```python
from build123d import *

# Parameters (mm, degrees)
SKETCH1_W                = 69
SKETCH1_H                = 45
BOSS_EXTRUDE1_DEPTH      = 10
BOSS_EXTRUDE2_DEPTH      = 12
BOSS_EXTRUDE2_DEPTH_BACK = 13
SKETCH5_R                = 19
SKETCH6_R                = 8
CUT_EXTRUDE1_DEPTH       = 146.555831213
FILLET1_R                = 25
FILLET2_R                = 15
FILLET3_R                = 5
FILLET4_R                = 2
FILLET5_R                = 25
FILLET6_R                = 30
SKETCH7_R                = 8
CUT_EXTRUDE2_DEPTH       = 138.282555338


with BuildPart() as part:
    # Sketch1 → Boss-Extrude1 (new body)
    with BuildSketch(Plane.XY):
        Rectangle(SKETCH1_W, SKETCH1_H)
    extrude(amount=BOSS_EXTRUDE1_DEPTH)

    # Sweep1: sweep along a path in Sketch3
    with BuildLine(Plane(origin=(15.5, 0, 0), x_dir=(0, 0, -1), z_dir=(1, 0, 0))) as sweep1_path:
        Line((-10, -22.5), (-100, -22.5))
        Line((-100, -22.5), (-100, -52.5))
    # Sketch4 → Sweep1 (sweep)
    with BuildSketch(Plane.XY.offset(10)):
        Polygon((34.5, -22.5), (-3.5, -22.5), (-3.5, -12.5), (10.5, -12.5), (10.5, -2.5), (20.5, -2.5), (20.5, -12.5), (34.5, -12.5), align=None)
    sweep(path=sweep1_path.line, transition=Transition.RIGHT)

    # Sketch5 → Boss-Extrude2 (add, two sides: drawn at the far end of the back side and taken through both)
    with BuildSketch(Plane.XY.offset(110).offset(-BOSS_EXTRUDE2_DEPTH_BACK)):
        with Locations((15.5, -52.5)):
            Circle(SKETCH5_R)
    extrude(amount=BOSS_EXTRUDE2_DEPTH + BOSS_EXTRUDE2_DEPTH_BACK)

    # Sketch6 → Cut-Extrude1 (cut, through all)
    with BuildSketch(Plane.XY.offset(122)):
        with Locations((15.5, -52.5)):
            Circle(SKETCH6_R)
    extrude(amount=-CUT_EXTRUDE1_DEPTH, mode=Mode.SUBTRACT)

    # Fillet1
    fillet1_edges = [part.edges().sort_by_distance(p)[0] for p in [
        (15.5, -2.5, 120),
    ]]
    fillet(fillet1_edges, radius=FILLET1_R)

    # Fillet2
    fillet2_edges = [part.edges().sort_by_distance(p)[0] for p in [
        (3.5, -12.5, 110),
        (27.5, -12.5, 110),
    ]]
    fillet(fillet2_edges, radius=FILLET2_R)

    # Fillet3
    fillet3_edges = [part.edges().sort_by_distance(p)[0] for p in [
        (15.5, -22.5, 100),
    ]]
    fillet(fillet3_edges, radius=FILLET3_R)

    # Fillet4
    fillet4_edges = [part.edges().sort_by_distance(p)[0] for p in [
        (15.5, -33.5, 120),
    ]]
    fillet(fillet4_edges, radius=FILLET4_R - 0.0001)  # a hair under: the kernel refuses the full size

    # Fillet5
    fillet5_edges = [part.edges().sort_by_distance(p)[0] for p in [
        (15.5, -2.5, 10),
    ]]
    fillet(fillet5_edges, radius=FILLET5_R - 0.0001)  # a hair under: the kernel refuses the full size

    # Fillet6
    fillet6_edges = [part.edges().sort_by_distance(p)[0] for p in [
        (-3.5, -17.5, 10),
    ]]
    fillet(fillet6_edges, radius=FILLET6_R)

    # Sketch7 → Cut-Extrude2 (cut, through all)
    with BuildSketch(Plane.XY.offset(10)):
        with Locations((-12.5, 4.5)):
            Circle(SKETCH7_R)
    extrude(amount=-CUT_EXTRUDE2_DEPTH, mode=Mode.SUBTRACT)


solid = part.part
```
Part model, mm, in its own coordinate system. A direction names the side the tool comes from. Give positions to 0.01 mm unless a question says otherwise; leave off trailing zeros. Order: outer loops, then holes, each group sorted by start corner. A loop starts at its lowest first (then second) coordinate and runs counter-clockwise, first axis right, second up. Notation, with made-up numbers: (53, -3.75) - (78, -3.75) arc R21 ccw to (78, 18.25) - close; hole circle Ø2 at (56.5, 20.5). An arc over 180 degrees is marked (long way). Use one line per item in the form item = value.
Item 1: Pin check, flat tips, straight feed: pin 1 Ø9.5 at (x, y) = (15.5, -52.5) entering from -Z (3 decimals); pin 2 Ø17 at (y, z) = (0.5, 45.5) entering from -X; pin 3 Ø3.5 at (x, y) = (17.5, -29) entering from +Z; pin 4 Ø13.5 at (x, y) = (-9, 7.5) entering from +Z. Stop position of each tip, or through.
Solution:
pin_1 = through
pin_2 = 10.5
pin_3 = 120
pin_4 = 10
Item 2: Probe probe 1 along X at (y, z) = (4, 2); probe 2 along Y at (x, z) = (-12.5, 4.5); probe 3 along X at (y, z) = (-52, 107). List the from-to ranges inside material, lowest first. Write a range as from..to.
Solution:
probe_1 = -34.5..-20.48, -4.52..34.5
probe_2 = -22.5..-3.5, 12.5..22.5
probe_3 = -3.5..7.52, 23.48..34.5
Item 3: Which spindle directions (+Z, -Z, +X, -X, +Y, -Y) get a long thin tool onto all of the face, cutting with end or side? Do faces 1 (the face through (3, -12.5, 53)), 2 (the face through (-3.5, -22, 86)), 3 (the face through (0, 5, 10)). Say none if no direction does.
Solution:
face_1 = +Z, -X, +Y
face_2 = +Z, -X, +Y, -Y
face_3 = +Z, +Y
Item 4: Slice it at B-B on y = 4.5. Give the cut face in (x, z), and give its area (3 significant figures).
Solution:
outline = (-34.5, 0) - (-20.5, 0) - (-20.5, 10) - (-34.5, 10) - close; (-4.5, 0) - (34.5, 0) - (34.5, 10) - (20.5, 10) - (20.5, 17.65) - (10.5, 17.65) - (10.5, 10) - (-4.5, 10) - close
area = 607 mm2
Item 5: Two-plate mould, pull along Y, no slides. Class faces 4 (the face through (15, -32, 100)), 5 (the face through (16, -2.5, 65)), 6 (the face through (0, 0, 0)): released by +Y, released by -Y, zero draft, split by the parting line, or undercut.
Solution:
face_4 = undercut
face_5 = released by +Y
face_6 = zero draft
Item 6: Slice it at D-D on x = 26.5. Give the cut face in (y, z), and give its area (3 significant figures).
Solution:
outline = (-67.99, 97) - (-37.01, 97) - (-37.01, 100) - (-27.5, 100) arc R5 cw to (-22.5, 95) - (-22.5, 0) - (22.5, 0) - (22.5, 10) - (-12.5, 10) - (-12.5, 95) arc R15 ccw to (-27.5, 110) - (-37.01, 110) - (-37.01, 122) - (-67.99, 122) - close
area = 2,330 mm2
Item 7: Slice it at C-C on z = 82.5. Give the cut face in (x, y).
Solution:
outline = (-3.5, -22.5) - (34.5, -22.5) - (34.5, -12.5) - (20.5, -12.5) - (20.5, -2.5) - (10.5, -2.5) - (10.5, -12.5) - (-3.5, -12.5) - close
